The listing builds one solid part. Answer for the finished solid, in the listing's coordinates (mm). Face numbers are marked on the shaded views. A direction names the side the tool comes from. Round coordinates to 2 decimals unless told otherwise and drop trailing zeros. Loops run counter-clockwise (first coordinate to the right, second up) from the corner with the lowest first, then second, coordinate; pieces in that order, holes last. Notation, with made-up numbers: M 11,2.25 L 56,2.25 A27 ccw 56,22.25 Z; hole C 13,13 d8. An arc over 180 degrees is marked long. Put each result on its own line as item: value. Start each with the question number.
(1) Flat-ended cylindrical pins translate along their axes: P1, Ø6, axis at y = 0, z = 21, coming from the -X side; P2, Ø15, axis at x = 9, y = -2, coming from the +Z side. Find the tip coordinate at first contact, or state that the pin passes through.
(2) Determine the mould class of the marked faces 1, 2 and 3 for opening direction Z: released by +Z, released by -Z, zero draft, split by the parting line, or undercut.
(3) Section D-D, the plane y = -15.5 is taken. Determine the outline of the cut face in (x, z).
(4) Section B-B, the plane x = 10.1 is taken. Determine the outline of the cut face in (y, z), then the cut area to 3 significant figures.
(5) Section C-C, the plane y = 0 is taken. Determine the outline of the cut face in (x, z), then the cut area to 3 significant figures.
(6) Straight lines are drawn through the part: line 1 (Z direction, x = 13, y = 9); line 2 (Y direction, x = 10.1, z = 2.95); line 3 (X direction, y = -13, z = 39). For each, find the intervals that lie inside material, in ascending order.
(7) Which of the six approach directions +Z, -Z, +X, -X, +Y, -Y give full straight-line access (tool end or side, diameter ignored) to the marked faces 4 and 5?
(8) Section A-A, the plane z = 24.5 is taken. Determine the outline of the cut face in (x, y).
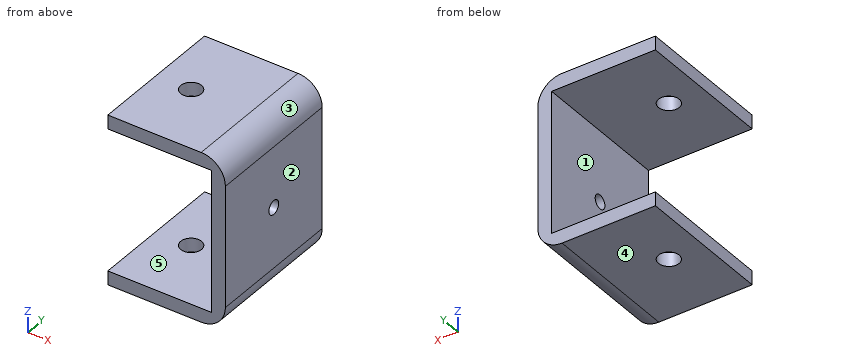
```python
from build123d import *

# Parameters (mm, degrees)
F1_DEPTH      = 20
F1_DEPTH_BACK = 20
F2_R          = 7
F3_R          = 2
F4_DEPTH      = 25
F5_R          = 3
F6_DEPTH      = 53


with BuildPart() as f1:
    # F0 (on Front) → F1 (new body, two sides)
    with BuildSketch(Plane.XZ) as f1_sk:
        Polygon((0, 4), (0, 0), (34, 0), (34, 49), (0, 49), (0, 45), (30, 45), (30, 4), align=None)
    extrude(amount=F1_DEPTH)
    extrude(f1_sk.sketch, amount=-F1_DEPTH_BACK)

    # F2
    f2_edges = [f1.edges().sort_by_distance(p)[0] for p in [
        (34, 0, 49),
        (34, 0, 0),
    ]]
    fillet(f2_edges, radius=F2_R)

    # F3 (on face) → F4 (cut)
    with BuildSketch(Plane.YZ.offset(34)):
        with Locations((0, 24.5)):
            Circle(F3_R)
    extrude(amount=-F4_DEPTH, mode=Mode.SUBTRACT)

    # F5 (on face) → F6 (cut)
    with BuildSketch(Plane.XY.offset(49)):
        with Locations((10.1, 0)):
            Circle(F5_R)
    extrude(amount=-F6_DEPTH, mode=Mode.SUBTRACT)


solid = f1.part
```
Recorded:
1. P1: stops at x = 30
1. P2: stops at z = 49
2. face 1: undercut
2. face 2: zero draft
2. face 3: released by +Z
3. outline: M 0,0 L 27,0 A7 ccw 34,7 L 34,42 A7 ccw 27,49 L 0,49 L 0,45 L 30,45 L 30,4 L 0,4 Z
4. outline: M -20,0 L -3,0 L -3,4 L -20,4 Z; M -20,45 L -3,45 L -3,49 L -20,49 Z; M 3,0 L 20,0 L 20,4 L 3,4 Z; M 3,45 L 20,45 L 20,49 L 3,49 Z
4. area: 272 mm²
5. outline: M 0,0 L 7.1,0 L 7.1,4 L 0,4 Z; M 0,45 L 7.1,45 L 7.1,49 L 0,49 Z; M 13.1,0 L 27,0 A7 ccw 34,7 L 34,22.5 L 30,22.5 L 30,4 L 13.1,4 Z; M 13.1,45 L 30,45 L 30,26.5 L 34,26.5 L 34,42 A7 ccw 27,49 L 13.1,49 Z
5. area: 351 mm²
6. line 1: z = 0 to 4, 45 to 49
6. line 2: y = -20 to -3, 3 to 20
6. line 3: x = 30 to 34
7. face 4: -Z, +X, -X, +Y, -Y
7. face 5: -X, +Y, -Y
8. outline: M 30,-20 L 34,-20 L 34,-2 L 30,-2 Z; M 30,2 L 34,2 L 34,20 L 30,20 Z
